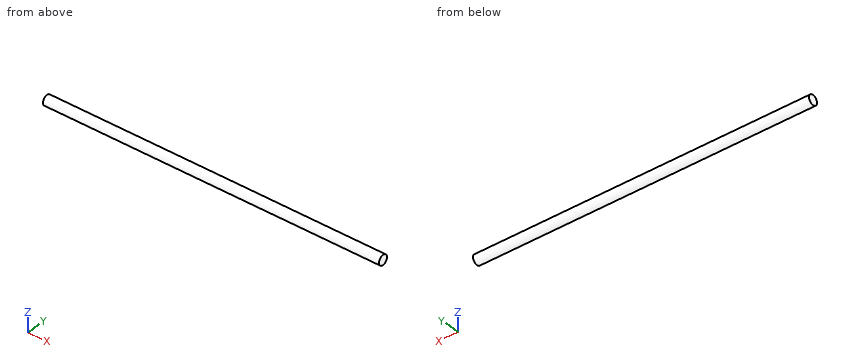
```python
from build123d import *

# Parameters (mm, degrees)
BOSS_EXTRUDE1_OUTLINE_R = 3.175
BOSS_EXTRUDE1_DEPTH     = 218.44


# Read off the part's stored shape, not the designer's step: Boss-Extrude1
with BuildPart() as part:
    # Boss-Extrude1 outline → Boss-Extrude1 (new body)
    with BuildSketch(Plane(origin=(-98.013718438, 0, 0), x_dir=(0, 0, -1), z_dir=(1, 0, 0))):
        with Locations((-21.267819308, -276.062087489)):
            Circle(BOSS_EXTRUDE1_OUTLINE_R)
    extrude(amount=BOSS_EXTRUDE1_DEPTH)


solid = part.part
```
Could you check a few things on this model? Use its own coordinates, in mm. Coordinates: 2 decimals unless noted, no trailing zeros. Order: outer loops, then holes, each group sorted by start corner. A loop starts at its lowest first (then second) coordinate and runs counter-clockwise, first axis right, second up. Notation, with made-up numbers: M 86.25,73 L 107.25,73 A13 ccw 107.25,88 Z; hole C 17.5,7 d2. An arc over 180 degrees is marked long. Use a Markdown table: item, result. Add a question column.
Q1. I want a section at A-A on y = -278.25. List the corners of the cut face in (x, z) for me, then the cut area to 3 significant figures.
Q2. I want a section at B-B on x = -6. List the corners of the cut face in (y, z) for me (3 decimals).
Q3. I'm going to push flat-ended pins straight in: pin 1 (1.5 mm diameter, centred on x = 11.5, y = -275, fed in from -Z); pin 2 (2 mm diameter, centred on x = -13.5, z = 20, fed in from +Y). Where does each tip first touch, or does it pass through?
Q4. If I drill on L1, parallel to Y at x = -42.5, z = 20.75; L2, parallel to Z at x = 83, y = -275.75; L3, parallel to Z at x = 110, y = -273.25, over which ranges is the centre line in solid material (lowest first)?
Q5. I want a section at C-C on z = 20. List the corners of the cut face in (x, y) for me.
Checked values:
| question | item | result |
|---|---|---|
| 1 | outline | M -98.01,18.97 L 120.43,18.97 L 120.43,23.57 L -98.01,23.57 Z |
| 1 | area | 1,010 mm² |
| 2 | outline | C -276.062,21.268 d6.35 |
| 3 | pin 1 | z = 18.11 |
| 3 | pin 2 | y = -272.9 |
| 4 | L1 | -279.19 to -272.93 |
| 4 | L2 | 18.11 to 24.43 |
| 4 | L3 | 19.79 to 22.74 |
| 5 | outline | M -98.01,-278.97 L 120.43,-278.97 L 120.43,-273.15 L -98.01,-273.15 Z |
